from build123d import *

# Parameters (mm, degrees)
SKETCH6_W           = 350
SKETCH6_H           = 350
SKETCH6_R           = 12.5
BOSS_EXTRUDE1_DEPTH = 5
SKETCH7_W           = 120
SKETCH7_H           = 350
BOSS_EXTRUDE2_DEPTH = 5
SKETCH8_R           = 2.5
CUT_EXTRUDE1_DEPTH  = 10


with BuildPart() as part:
    # Sketch6 → Boss-Extrude1 (new body)
    with BuildSketch(Plane(origin=(0, 0, 0), x_dir=(1, 0, 0), z_dir=(0, 1, 0))):
        Rectangle(SKETCH6_W, SKETCH6_H)
        with Locations(Location((0, 0, 0), (0, 0, 270))):
            Circle(SKETCH6_R, mode=Mode.SUBTRACT)
    extrude(amount=BOSS_EXTRUDE1_DEPTH)

    # Sketch7 → Boss-Extrude2 (add)
    with BuildSketch(Plane(origin=(0, 5, 0), x_dir=(1, 0, 0), z_dir=(0, 1, 0))):
        with Locations((-235, 0)):
            Rectangle(SKETCH7_W, SKETCH7_H)
    extrude(amount=-BOSS_EXTRUDE2_DEPTH)

    # Sketch8 → Cut-Extrude1 (cut)
    with BuildSketch(Plane(origin=(0, 5, 0), x_dir=(1, 0, 0), z_dir=(0, 1, 0))):
        with Locations(Location((-287.5, -43.500000153, 0), (0, 0, 270))):
            Circle(SKETCH8_R)
        with Locations(Location((-287.5, -68.500000153, 0), (0, 0, 270))):
            Circle(SKETCH8_R)
        with Locations(Location((-287.5, 68.500000153, 0), (0, 0, 270))):
            Circle(SKETCH8_R)
        with Locations(Location((-287.5, 43.500000153, 0), (0, 0, 270))):
            Circle(SKETCH8_R)
    extrude(amount=-CUT_EXTRUDE1_DEPTH, mode=Mode.SUBTRACT)


solid = part.part
Can you work these out from the model? Positions are in its coordinate system, mm. Give positions to 0.01 mm unless a question says otherwise; leave off trailing zeros. Loops run counter-clockwise (first coordinate to the right, second up) from the corner with the lowest first, then second, coordinate; pieces in that order, holes last. Notation, with made-up numbers: (60, 74.25) -> (66, 74.25) arc R29 ccw to (66, 95.25) -> close; hole circle Ø3 at (19, -0.75). An arc over 180 degrees is marked (long way). Use one line per item in the form item = value.
1) I need wall thicknesses on line 1 along Z through (x, y) = (-287.5, 1.65); line 2 along X through (y, z) = (2.7, 43.5); line 3 along X through (y, z) = (1.1, 0). Which ranges of each line are inside material? Lowest first, please.
Answers:
line_1 = -175 to -71, -66 to -46, -41 to 41, 46 to 66, 71 to 175
line_2 = -295 to -290, -285 to 175
line_3 = -295 to -12.5, 12.5 to 175
2) We'd pull the mould along Z, two halves only. Please class faces 1 (the face through (-63, 5, -2)), 2 (the face through (3.755, 2.465, 11.923)): released by +Z, released by -Z, zero draft, split by the parting line, or undercut.
Answers:
face_1 = zero draft
face_2 = undercut
3) Will these pins go through, and if not, where does the flat tip stop? pin 1 (1.5 mm diameter, centred on x = -26, z = 130, fed in from -Y); pin 2 (4 mm diameter, centred on x = -287.5, z = -68.5, fed in from -Y).
Answers:
pin_1 = 0
pin_2 = through
4) If we section it at A-A (z = 0): Please give me the cut outline in (x, y).
Answers:
outline = (-295, 0) -> (-12.5, 0) -> (-12.5, 5) -> (-295, 5) -> close; (12.5, 0) -> (175, 0) -> (175, 5) -> (12.5, 5) -> close
